Input: part model. Units: mm. Frame: model coordinates. A direction names the side the tool comes from. Round coordinates to 2 decimals unless told otherwise and drop trailing zeros. Write each loop counter-clockwise with the first axis right and the second up, starting at its lowest first coordinate (ties: lowest second). Pieces come first, ordered by that corner, then holes. Notation, with made-up numbers: (82.25, 12) - (124.25, 12) arc R24 ccw to (124.25, 39) - close; hole circle Ø1 at (16, -0.5). An arc over 180 degrees is marked (long way). Use one line per item in the form item = value.
```python
from build123d import *

# Parameters (mm, degrees)
F0_W     = 300
F0_H     = 300
F1_DEPTH = 20
F2_W     = 150
F2_H     = 150
F3_DEPTH = 50


with BuildPart() as f1:
    # F0 (on Top) → F1 (new body, symmetric)
    with BuildSketch(Plane.XY):
        with Locations((-4.049069, -3.999319)):
            Rectangle(F0_W, F0_H)
    extrude(amount=F1_DEPTH, both=True)

    # F2 (on face) → F3 (cut)
    with BuildSketch(Plane.XY.offset(20)):
        with Locations((0.162162, 0.858896)):
            Rectangle(F2_W, F2_H)
    extrude(amount=-F3_DEPTH, mode=Mode.SUBTRACT)


solid = f1.part
```
(1) Cut plane C-C on z = 8. Output: boundary loops of the cut face in (x, y), then the cut area to 3 significant figures.
Derived:
outline = (-154.05, -154) - (145.95, -154) - (145.95, 146) - (-154.05, 146) - close; hole (-74.84, -74.14) - (75.16, -74.14) - (75.16, 75.86) - (-74.84, 75.86) - close
area = 67,500 mm^2
(2) Draft query along X for faces 3 (the face through (-74.838, 0, 0)), 4 (the face through (-106, -2, 20)), 5 (the face through (145.951, -6, 0)), 6 (the face through (75.162, 0, 0)). Return one class per face: released by +X, released by -X, zero draft, split by the parting line, or undercut.
Derived:
face_3 = undercut
face_4 = zero draft
face_5 = released by +X
face_6 = undercut
(3) Access query for faces 1 (the face through (-1, 75.859, 0)), 2 (the face through (-6, -153.999, 0)). Directions: +Z, -Z, +X, -X, +Y, -Y. A direction counts if a zero-diameter tool reaches every point of the face in a straight line with its end or side. Return the directions, or none.
Derived:
face_1 = +Z, -Z
face_2 = +Z, -Z, +X, -X, -Y
(4) Material intervals for L1, parallel to X at y = -38.5, z = -12; L2, parallel to Y at x = -0.5, z = 0.5, sorted ascending.
Derived:
L1 = -154.05 to -74.84, 75.16 to 145.95
L2 = -154 to -74.14, 75.86 to 146
(5) Cut plane A-A on y = -51. Output: boundary loops of the cut face in (x, z), then the cut area to 3 significant figures.
Derived:
outline = (-154.05, -20) - (-74.84, -20) - (-74.84, 20) - (-154.05, 20) - close; (75.16, -20) - (145.95, -20) - (145.95, 20) - (75.16, 20) - close
area = 6,000 mm^2
(6) Cut plane B-B on x = -17. Output: boundary loops of the cut face in (y, z).
Derived:
outline = (-154, -20) - (-74.14, -20) - (-74.14, 20) - (-154, 20) - close; (75.86, -20) - (146, -20) - (146, 20) - (75.86, 20) - close
